from build123d import *

# Parameters (mm, degrees)
SKETCH24_W              = 19.01040764
SKETCH24_H              = 82.93150469
SKETCH24_W_2            = 50
SKETCH24_H_2            = 120.95231997
BOSS_EXTRUDE1_DEPTH     = 2
SKETCH25_W              = 51.01040764
SKETCH25_H              = 134.95231997
BOSS_EXTRUDE2_DEPTH     = 5
CUT_EXTRUDE2_DEPTH      = 303.633154318
CUT_EXTRUDE2_DEPTH_BACK = 303.633154318
SKETCH24_3_W            = 19.01040764
SKETCH24_3_H            = 82.93150469
SKETCH24_3_W_2          = 50
SKETCH24_3_H_2          = 120.95231997
CUT_EXTRUDE3_DEPTH      = 3
FILLET1_R               = 12
SKETCH28_R              = 3
CUT_EXTRUDE4_DEPTH      = 150.018673002
FILLET2_R               = 5


with BuildPart() as part:
    # Sketch24 → Boss-Extrude1 (new body)
    with BuildSketch(Plane.XY):
        with Locations((20.91706823, 70.762534541)):
            Rectangle(SKETCH24_W, SKETCH24_H)
        with Locations((55.42227205, 70.762534541)):
            Rectangle(SKETCH24_W_2, SKETCH24_H_2)
        Polygon((250.158478802, 10.286374556), (250.158478802, 29.296782196), (250.158478802, 112.228286886), (250.158478802, 131.238694526), (200.158478802, 131.238694526), (200.158478802, 10.286374556), align=None)
        with Locations((259.663682622, 70.762534541)):
            Rectangle(SKETCH24_W, SKETCH24_H)
    extrude(amount=-BOSS_EXTRUDE1_DEPTH)

    # Sketch25 → Boss-Extrude2 (add)
    with BuildSketch(Plane.XY):
        with Locations((29.91706823, 70.762534541)):
            Rectangle(SKETCH25_W, SKETCH25_H)
    extrude(amount=BOSS_EXTRUDE2_DEPTH)

    # Sketch24<3> → Cut-Extrude2 (cut, two sides: drawn at the far end of the back side and taken through both)
    with BuildSketch(Plane.XY.offset(-CUT_EXTRUDE2_DEPTH_BACK)):
        with Locations((20.91706823, 70.762534541)):
            Rectangle(SKETCH24_3_W, SKETCH24_3_H)
        with Locations((55.42227205, 70.762534541)):
            Rectangle(SKETCH24_3_W_2, SKETCH24_3_H_2)
        Polygon((250.158478802, 10.286374556), (250.158478802, 29.296782196), (250.158478802, 112.228286886), (250.158478802, 131.238694526), (200.158478802, 131.238694526), (200.158478802, 10.286374556), align=None)
        with Locations((259.663682622, 70.762534541)):
            Rectangle(SKETCH24_3_W, SKETCH24_3_H)
    extrude(amount=CUT_EXTRUDE2_DEPTH + CUT_EXTRUDE2_DEPTH_BACK, mode=Mode.SUBTRACT)

    # Sketch2 → Cut-Extrude3 (cut)
    with BuildSketch(Plane.XY):
        with BuildLine():
            Line((16.41186441, 136.238694526), (264.168886442, 136.238694526))
            ThreePointArc((264.168886442, 136.238694526), (271.239954254, 133.309762338), (274.168886442, 126.238694526))
            Line((274.168886442, 126.238694526), (274.168886442, 15.286374556))
            ThreePointArc((274.168886442, 15.286374556), (271.239954254, 8.215306744), (264.168886442, 5.286374556))
            Line((264.168886442, 5.286374556), (16.41186441, 5.286374556))
            ThreePointArc((16.41186441, 5.286374556), (9.340796598, 8.215306744), (6.41186441, 15.286374556))
            Line((6.41186441, 15.286374556), (6.41186441, 126.238694526))
            ThreePointArc((6.41186441, 126.238694526), (9.340796598, 133.309762338), (16.41186441, 136.238694526))
        make_face()
    extrude(amount=CUT_EXTRUDE3_DEPTH, mode=Mode.SUBTRACT)

    # Fillet1
    fillet1_edges = [part.edges().sort_by_distance(p)[0] for p in [
        (4.41186441, 138.238694526, 2.5),
        (4.41186441, 3.286374556, 2.5),
    ]]
    fillet(fillet1_edges, radius=FILLET1_R)

    # Sketch28 → Cut-Extrude4 (cut, through all)
    with BuildSketch(Plane.XY):
        with Locations((25.42227205, 117.228286886)):
            Circle(SKETCH28_R)
        with Locations((16.41186441, 15.286374556)):
            Circle(SKETCH28_R)
        with Locations((16.41186441, 117.228286886)):
            Circle(SKETCH28_R)
        with Locations((25.42227205, 15.286374556)):
            Circle(SKETCH28_R)
        with Locations((25.42227205, 24.296782196)):
            Circle(SKETCH28_R)
        with Locations((16.41186441, 24.296782196)):
            Circle(SKETCH28_R)
        with Locations((25.42227205, 126.238694526)):
            Circle(SKETCH28_R)
        with Locations((16.41186441, 126.238694526)):
            Circle(SKETCH28_R)
    extrude(amount=CUT_EXTRUDE4_DEPTH, mode=Mode.SUBTRACT)

    # Fillet2
    fillet2_edges = [part.edges().sort_by_distance(p)[0] for p in [
        (30.42227205, 29.296782196, 4),
        (30.42227205, 112.228286886, 4),
    ]]
    fillet(fillet2_edges, radius=FILLET2_R)


solid = part.part
Read the model definition and answer for the solid it produces. Units are mm, in the model's axes. A direction names the side the tool comes from. Coordinates: 2 decimals unless noted, no trailing zeros. Loops run counter-clockwise (first coordinate to the right, second up) from the corner with the lowest first, then second, coordinate; pieces in that order, holes last. Notation, with made-up numbers: (31, 27) - (64, 27) arc R6 ccw to (64, 35) - close; hole circle Ø7 at (0, 41). An arc over 180 degrees is marked (long way). Answer in a Markdown table with one row per item.
Q1. For faces 4 (the flat face through (6.412, 70, 1)), 5 (the flat face through (5, 71, 0)), 6 (the cylindrical face through (29, 27.79, 4.01)), determine the directions among +Z, -Z, +X, -X, +Y, -Y from which every point of the face is accessible in a straight line to the end or side of a thin tool.
Here are the results:
| item | result |
|---|---|
| face 4 | -Z, +X |
| face 5 | -Z, +X, -X, +Y, -Y |
| face 6 | +Z, -Z, +X |
Q2. Find section B-B on z = 3.8. Count the separate pieces of the cut face and the enclosed holes in it, plus the area to 3 significant figures.
Here are the results:
| item | result |
|---|---|
| separate pieces | 1 |
| enclosed holes | 8 |
| area | 1,980 mm^2 |
Q3. Straight lines are drawn through the part: line 1 along X through (y, z) = (126.5, 4.75); line 2 along Y through (x, z) = (44, 4.1); line 3 along Y through (x, z) = (40, 2). For each, find the intervals that lie inside material, in ascending order. Write a range as [from, to].
Here are the results:
| item | result |
|---|---|
| line 1 | x = [4.41, 13.42], [19.4, 22.43], [28.41, 30.42] |
| line 2 | y = [3.29, 10.29], [131.24, 138.24] |
| line 3 | y = [3.29, 5.29], [136.24, 138.24] |
Q4. The mould has two halves that part along Y. Classify faces 1 (the cylindrical face through (7.834, 134.63, 2.535)), 2 (the cylindrical face through (15.8, 123.3, 4)), 3 (the flat face through (11, 66, 5)): pulls with the +Y half, pulls with the -Y half, needs draft (parallel to the pull), parting line crosses it, or undercut.
Here are the results:
| item | result |
|---|---|
| face 1 | pulls with the +Y half |
| face 2 | undercut |
| face 3 | needs draft |
Q5. Find section A-A on x = 43.5. Write down the section's boundary in (y, z).
Here are the results:
| item | result |
|---|---|
| outline | (3.29, 0) - (5.29, 0) - (5.29, 3) - (10.29, 3) - (10.29, 5) - (3.29, 5) - close; (131.24, 3) - (136.24, 3) - (136.24, 0) - (138.24, 0) - (138.24, 5) - (131.24, 5) - close |
Q6. Given P1, Ø0.6, axis at y = 65.5, z = 3.5, coming from the +X side; P2, Ø8, axis at x = 25.42, y = 15.29, coming from the -Z side; P3, Ø2, axis at y = 14.5, z = 3.5, coming from the +X side, each flat-ended and moving along its own axis, determine where each tip first touches the part or whether it passes through.
Here are the results:
| item | result |
|---|---|
| P1 | stops at x = 11.41 |
| P2 | stops at z = 3 |
| P3 | stops at x = 30.42 |
Q7. Find section C-C on y = 124.5. Write down the section's boundary in (x, z).
Here are the results:
| item | result |
|---|---|
| outline | (4.41, 0) - (6.41, 0) - (6.41, 3) - (13.97, 3) - (13.97, 5) - (4.41, 5) - close; (18.86, 3) - (22.98, 3) - (22.98, 5) - (18.86, 5) - close; (27.87, 3) - (30.42, 3) - (30.42, 5) - (27.87, 5) - close |
Q8. Find section D-D on y = 42.5. Write down the section's boundary in (x, z), plus the area to 3 significant figures.
Here are the results:
| item | result |
|---|---|
| outline | (4.41, 0) - (6.41, 0) - (6.41, 3) - (11.41, 3) - (11.41, 5) - (4.41, 5) - close |
| area | 20.0 mm^2 |
